from build123d import *

# Parameters (mm, degrees)
SKETCH_1_W          = 14
SKETCH_1_H          = 20
SKETCH_2_R          = 2
CUT_EXTRUDE_1_DEPTH = 130.539569244


with BuildPart() as part:
    # 草图1 → 旋转1 (revolve)
    with BuildSketch(Plane.XY, mode=Mode.PRIVATE) as revolve_1_sk:
        with Locations((83.5, 10)):
            Rectangle(SKETCH_1_W, SKETCH_1_H)
    revolve(revolve_1_sk.sketch.rotate(Axis((0, 0, 0), (0, 1, 0)), 90), axis=Axis((0, 0, 0), (0, 1, 0)))

    # 草图2 → 切除-拉伸1 (cut, through all)
    with BuildSketch(Plane(origin=(0, 20, 0), x_dir=(1, 0, 0), z_dir=(0, 1, 0))):
        with Locations(Location((-83.9, 0, 0), (0, 0, 270))):
            Circle(SKETCH_2_R)
        with Locations(Location((-59.326258942, 59.326258942, 0), (0, 0, 270))):
            Circle(SKETCH_2_R)
        with Locations(Location((0, 83.9, 0), (0, 0, 270))):
            Circle(SKETCH_2_R)
        with Locations(Location((59.326258942, 59.326258942, 0), (0, 0, 270))):
            Circle(SKETCH_2_R)
        with Locations(Location((83.9, 0, 0), (0, 0, 270))):
            Circle(SKETCH_2_R)
        with Locations(Location((59.326258942, -59.326258942, 0), (0, 0, 270))):
            Circle(SKETCH_2_R)
        with Locations(Location((0, -83.9, 0), (0, 0, 270))):
            Circle(SKETCH_2_R)
        with Locations(Location((-59.326258942, -59.326258942, 0), (0, 0, 270))):
            Circle(SKETCH_2_R)
    extrude(amount=-CUT_EXTRUDE_1_DEPTH, mode=Mode.SUBTRACT)


solid = part.part
Read the model definition and answer for the solid it produces. Units are mm, in the model's axes. Coordinates: 2 decimals unless noted, no trailing zeros. Order: outer loops, then holes, each group sorted by start corner. A loop starts at its lowest first (then second) coordinate and runs counter-clockwise, first axis right, second up. Notation, with made-up numbers: (73.5, -24.5) - (108.5, -24.5) arc R23 cw to (108.5, 12.5) - close; hole circle Ø5 at (-22, 33.5). An arc over 180 degrees is marked (long way). Use one line per item in the form item = value.
(1) For a pull along Z with two mould halves and no side action, classify faces 1 (the face through (-57.343, 10.14, -59.587)), 2 (the face through (47, 20, -61)), 3 (the face through (-27.18, 10.14, -86.32)) as pulls with the +Z half, pulls with the -Z half, needs draft (parallel to the pull), parting line crosses it, or undercut.
Computed values:
face_1 = undercut
face_2 = needs draft
face_3 = parting line crosses it
(2) Given pin 1 Ø12 at (x, y) = (39.5, 17.5) entering from +Z; pin 2 Ø1.5 at (y, z) = (5.5, 14.5) entering from +X; pin 3 Ø6 at (y, z) = (9.5, 39) entering from -X, each flat-ended and moving along its own axis, determine where each tip first touches the part or whether it passes through.
Computed values:
pin_1 = 84.07
pin_2 = 89.45
pin_3 = -83.03
(3) Section B-B, the plane x = -12 is taken. Give the vertices of the cut face in (y, z).
Computed values:
outline = (0, -89.7) - (20, -89.7) - (20, -75.55) - (0, -75.55) - close; (0, 75.55) - (20, 75.55) - (20, 89.7) - (0, 89.7) - close
(4) Section C-C, the plane y = 13.25 is taken. Give the number of separate pieces and of enclosed holes in the cut face, then the cut area to 3 significant figures.
Computed values:
separate_pieces = 1
enclosed_holes = 9
area = 7,240 mm²
(5) Straight lines are drawn through the part: L1, parallel to X at y = 14, z = 0; L2, parallel to X at y = 18.25, z = 58.5; L3, parallel to X at y = 15, z = 15.5. For each, find the intervals that lie inside material, in ascending order.
Computed values:
L1 = -90.5 to -85.9, -81.9 to -76.5, 76.5 to 81.9, 85.9 to 90.5
L2 = -69.05 to -61.15, -57.5 to -49.3, 49.3 to 57.5, 61.15 to 69.05
L3 = -89.16 to -74.91, 74.91 to 89.16
(6) Section A-A, the plane z = -26.5 is taken. Give the vertices of the cut face in (x, y), then the cut area to 3 significant figures.
Computed values:
outline = (-86.53, 0) - (-71.76, 0) - (-71.76, 20) - (-86.53, 20) - close; (71.76, 0) - (86.53, 0) - (86.53, 20) - (71.76, 20) - close
area = 591 mm²
